from build123d import *

# Parameters (mm, degrees)
BOSS_EXTRUDE1_DEPTH     = 1.5875
M5_CLEARANCE_HOLE1_D    = 5.5
SKETCH11_W              = 91
SKETCH11_H              = 18.5
CUT_EXTRUDE1_DEPTH      = 1
CUT_EXTRUDE1_DEPTH_BACK = 2.5875
M4_CLEARANCE_HOLE1_D    = 4.5
FILLET1_R               = 3
SKETCH15_W              = 20.5
SKETCH15_H              = 210
CUT_EXTRUDE2_DEPTH      = 1
CUT_EXTRUDE2_DEPTH_BACK = 2.5875


with BuildPart() as part:
    # Sketch1 → Boss-Extrude1 (new body)
    with BuildSketch(Plane(origin=(0, 0, 0), x_dir=(1, 0, 0), z_dir=(0, 1, 0))):
        Polygon((91.75, -187.647941311), (-208.25, -187.647941311), (-208.25, 92.973423913), (-208.25, 125.872458689), (-126.25, 125.872458689), (-126.25, 192.372458689), (-117.25, 192.372458689), (176.75, 192.372458689), (176.75, 157.382658689), (211.75, 157.382658689), (211.75, -157.627541311), (211.75, -187.647941311), align=None)
    extrude(amount=BOSS_EXTRUDE1_DEPTH)

    # M5 Clearance Hole1 (through all)
    with Locations(Plane(origin=(0, 1.5875, 0), x_dir=(1, 0, 0), z_dir=(0, 1, 0))):
        with Locations((-153.937540098, -177.647941311), (-135.677540098, -177.647941311), (-117.417540098, -177.647941311), (117.417540098, -177.647941311), (135.677540098, -177.647941311), (153.937540098, -177.647941311)):
            Hole(M5_CLEARANCE_HOLE1_D / 2)

    # Sketch11 → Cut-Extrude1 (cut, two sides)
    with BuildSketch(Plane(origin=(0, 1.5875, 0), x_dir=(1, 0, 0), z_dir=(0, 1, 0))) as cut_extrude1_sk:
        with Locations((131.25, 183.122458689)):
            Rectangle(SKETCH11_W, SKETCH11_H)
    extrude(amount=CUT_EXTRUDE1_DEPTH, mode=Mode.SUBTRACT)
    extrude(cut_extrude1_sk.sketch, amount=-CUT_EXTRUDE1_DEPTH_BACK, mode=Mode.SUBTRACT)

    # M4 Clearance Hole1 (through all)
    with Locations(Plane(origin=(0, 1.5875, 0), x_dir=(1, 0, 0), z_dir=(0, 1, 0))):
        with Locations((96.75, 163.872458689), (166.75, 163.872458689)):
            Hole(M4_CLEARANCE_HOLE1_D / 2)

    # Fillet1
    fillet1_edges = [part.edges().sort_by_distance(p)[0] for p in [
        (211.75, 0.79375, 187.647941311),
        (-208.25, 0.79375, 187.647941311),
        (-208.25, 0.79375, -125.872458689),
        (-126.25, 0.79375, -125.872458689),
        (-126.25, 0.79375, -192.372458689),
        (176.75, 0.79375, -157.382658689),
        (211.75, 0.79375, -157.382658689),
        (176.75, 0.79375, -173.872458689),
        (85.75, 0.79375, -173.872458689),
        (85.75, 0.79375, -192.372458689),
    ]]
    fillet(fillet1_edges, radius=FILLET1_R)

    # Sketch15 → Cut-Extrude2 (cut, two sides)
    with BuildSketch(Plane(origin=(0, 1.5875, 0), x_dir=(1, 0, 0), z_dir=(0, 1, 0))) as cut_extrude2_sk:
        with Locations((-198, -42.647941311)):
            Rectangle(SKETCH15_W, SKETCH15_H)
        with Locations((201.5, -42.647941311)):
            Rectangle(SKETCH15_W, SKETCH15_H)
    extrude(amount=CUT_EXTRUDE2_DEPTH, mode=Mode.SUBTRACT)
    extrude(cut_extrude2_sk.sketch, amount=-CUT_EXTRUDE2_DEPTH_BACK, mode=Mode.SUBTRACT)


solid = part.part
CAD build for the part. Positions are in the model's coordinates, mm. Round coordinates to 2 decimals unless told otherwise and drop trailing zeros. Loops run counter-clockwise (first coordinate to the right, second up) from the corner with the lowest first, then second, coordinate; pieces in that order, holes last.
(1) Cut at A-A (z = 134.5). Give the cut face in (x, y), plus the area to 3 significant figures.
(2) Drop flat-ended pins along their axis: pin 1 (0.8 mm diameter, centred on y = 1, z = 8.5, fed in from -X); pin 2 (0.8 mm diameter, centred on y = 1, z = -180, fed in from +X); pin 3 (4.5 mm diameter, centred on x = 117.42, z = 177.65, fed in from -Y); pin 4 (0.8 mm diameter, centred on y = 1, z = -161.5, fed in from -X). Give the stop position or say it passes through.
(3) Wall check: line 1 along Z through (x, y) = (-190, 1); line 2 along Z through (x, y) = (-154, 0.6); line 3 along X through (y, z) = (0.55, -36). Give the ranges that are in metal, low to high.
(4) Cut at B-B (y = 0.5). State how many separate pieces and enclosed holes the cut face has, plus the area to 3 significant figures.
(5) Cut at C-C (z = -138). Give the cut face in (x, y).
Findings below:
1. outline: (-187.75, 0) - (191.25, 0) - (191.25, 1.59) - (-187.75, 1.59) - close
1. area: 602 mm2
2. pin 1: stops at x = -187.75
2. pin 2: stops at x = 85.75
2. pin 3: passes through
2. pin 4: stops at x = -126.25
3. line 1: z = -125.87 to -62.35, 147.65 to 187.65
3. line 2: z = -125.87 to 174.9, 180.4 to 187.65
3. line 3: x = -187.75 to 191.25
4. separate pieces: 1
4. enclosed holes: 8
4. area: 142,000 mm2
5. outline: (-126.25, 0) - (211.75, 0) - (211.75, 1.59) - (-126.25, 1.59) - close
